For this review, take the finished solid that the model builds, in its own axes (mm). Face numbers are marked on the shaded views. A direction names the side the tool comes from. Give positions to 0.01 mm unless a question says otherwise; leave off trailing zeros. Order: outer loops, then holes, each group sorted by start corner. A loop starts at its lowest first (then second) coordinate and runs counter-clockwise, first axis right, second up.
from build123d import *

# Parameters (mm, degrees)
F1_DEPTH = 25
F2_W     = 11.483927
F2_H     = 17.204142
F3_DEPTH = 76.6


with BuildPart() as f1:
    # F0 (on Front) → F1 (new body)
    with BuildSketch(Plane.XZ):
        Polygon((-60, 10), (-60, 0), (-20, 0), (-20, 20), (20, 20), (20, 0), (60, 0), (60, 10), (35, 10), (35, 50), (15, 50), (15, 40), (-15, 40), (-15, 50), (-35, 50), (-35, 10), align=None)
    extrude(amount=F1_DEPTH)

    # F2 (on face) → F3 (cut)
    with BuildSketch(Plane(origin=(-35, 0, 0), x_dir=(0, -1, 0), z_dir=(-1, 0, 0))):
        with Locations((12.402802, 41.397929)):
            Rectangle(F2_W, F2_H)
    extrude(amount=-F3_DEPTH, mode=Mode.SUBTRACT)


solid = f1.part
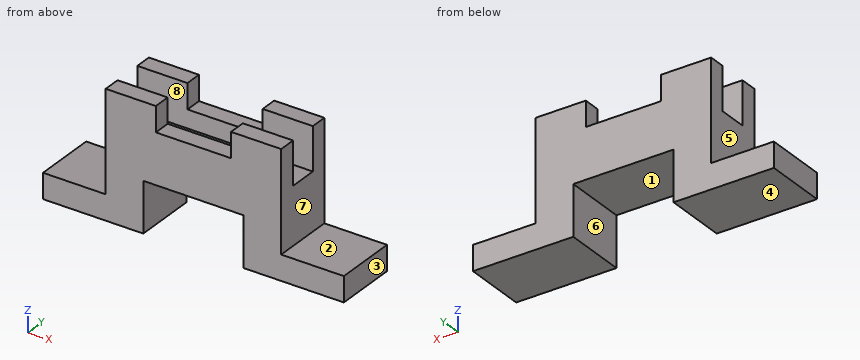
1) Clearance check with flat-ended pins moving along their axes: pin 1 (7.5 mm diameter, centred on x = -2, y = -17, fed in from -Z); pin 2 (12.5 mm diameter, centred on y = -7.5, z = 36, fed in from -X); pin 3 (1 mm diameter, centred on x = -4.5, y = -12, fed in from +Z). State where each tip first meets the part, or that it passes through.
Answer sheet:
pin 1: stops at z = 20
pin 2: stops at x = -35
pin 3: stops at z = 32.8
2) We need section B-B on z = 41.5. Give the boundary of the cut face in (x, y), then the cut area to 3 significant figures.
Answer sheet:
outline: (-35, -25) - (-15, -25) - (-15, -18.14) - (-35, -18.14) - close; (-35, -6.66) - (-15, -6.66) - (-15, 0) - (-35, 0) - close; (15, -25) - (35, -25) - (35, -18.14) - (15, -18.14) - close; (15, -6.66) - (35, -6.66) - (35, 0) - (15, 0) - close
area: 541 mm2
3) We need section A-A on z = 36.5. Give the boundary of the cut face in (x, y), then the cut area to 3 significant figures.
Answer sheet:
outline: (-35, -25) - (35, -25) - (35, -18.14) - (-35, -18.14) - close; (-35, -6.66) - (35, -6.66) - (35, 0) - (-35, 0) - close
area: 946 mm2
4) We need section C-C on y = -16.5. Give the boundary of the cut face in (x, z).
Answer sheet:
outline: (-60, 0) - (-20, 0) - (-20, 20) - (20, 20) - (20, 0) - (60, 0) - (60, 10) - (35, 10) - (35, 32.8) - (-35, 32.8) - (-35, 10) - (-60, 10) - close
5) Tool access review of the marked faces 4, 5, 6, 7 and 8: name each direction out of +Z, -Z, +X, -X, +Y, -Y from which nothing blocks a thin tool from reaching the whole face with its end or side.
Answer sheet:
face 4: -Z, +X, -X, +Y, -Y
face 5: +Z, -X, +Y, -Y
face 6: -Z, +Y, -Y
face 7: +Z, +X, +Y, -Y
face 8: +Z, +X, -X
6) Draft analysis for pull direction X (two halves, no side actions). For the marked faces 1, 2 and 3, state which applies: +X half, -X half, draft (parallel to the pull), parting line (faces both ways), or undercut.
Answer sheet:
face 1: undercut
face 2: draft
face 3: +X half
7) We need section D-D on x = 31.5. Give the boundary of the cut face in (y, z), then the cut area to 3 significant figures.
Answer sheet:
outline: (-25, 0) - (0, 0) - (0, 50) - (-6.66, 50) - (-6.66, 32.8) - (-18.14, 32.8) - (-18.14, 50) - (-25, 50) - close
area: 1,050 mm2
8) To check wall thickness, follow line 1 (X direction, y = -2.25, z = 3.5); line 2 (X direction, y = -3, z = 43.5); line 3 (X direction, y = -21, z = 25.5). State the ranges of each line that lie inside material, in increasing order.
Answer sheet:
line 1: x = -60 to -20, 20 to 60
line 2: x = -35 to -15, 15 to 35
line 3: x = -35 to 35
